```python
from build123d import *

# Parameters (mm, degrees)
F1_DEPTH = 0.3


with BuildPart() as f1:
    # F0 (on Top) → F1 (new body)
    with BuildSketch(Plane.XY):
        with BuildLine():
            ThreePointArc((68.445332, -5.526652), (68.785509, -6.832291), (68.9, -8.176652))
            Line((68.9, -8.176652), (102.9, -8.176652))
            Line((102.9, -8.176652), (102.9, 8.323348))
            Line((102.9, 8.323348), (87.9, 8.323348))
            ThreePointArc((87.9, 8.323348), (87.785509, 6.978988), (87.445332, 5.673348))
            ThreePointArc((87.445332, 5.673348), (79.95, 0.373348), (72.454668, 5.673348))
            ThreePointArc((72.454668, 5.673348), (72.114491, 6.978988), (72, 8.323348))
            Line((72, 8.323348), (49.9, 8.323348))
            ThreePointArc((49.9, 8.323348), (49.785509, 6.978988), (49.445332, 5.673348))
            ThreePointArc((49.445332, 5.673348), (41.95, 0.373348), (34.454668, 5.673348))
            ThreePointArc((34.454668, 5.673348), (34.114491, 6.978988), (34, 8.323348))
            Line((34, 8.323348), (0, 8.323348))
            Line((0, 8.323348), (0, -8.176652))
            Line((0, -8.176652), (15, -8.176652))
            ThreePointArc((15, -8.176652), (15.114491, -6.832291), (15.454668, -5.526652))
            ThreePointArc((15.454668, -5.526652), (22.95, -0.226652), (30.445332, -5.526652))
            ThreePointArc((30.445332, -5.526652), (30.785509, -6.832291), (30.9, -8.176652))
            Line((30.9, -8.176652), (53, -8.176652))
            ThreePointArc((53, -8.176652), (53.114491, -6.832291), (53.454668, -5.526652))
            ThreePointArc((53.454668, -5.526652), (60.95, -0.226652), (68.445332, -5.526652))
        make_face()
        with BuildLine():
            Line((15.454668, -5.526652), (30.445332, -5.526652))
            ThreePointArc((30.445332, -5.526652), (22.95, -0.226652), (15.454668, -5.526652))
        make_face()
        with BuildLine():
            ThreePointArc((34.454668, 5.673348), (41.95, 0.373348), (49.445332, 5.673348))
            Line((49.445332, 5.673348), (34.454668, 5.673348))
        make_face()
        with BuildLine():
            Line((53.454668, -5.526652), (68.445332, -5.526652))
            ThreePointArc((68.445332, -5.526652), (60.95, -0.226652), (53.454668, -5.526652))
        make_face()
        with BuildLine():
            ThreePointArc((72.454668, 5.673348), (79.95, 0.373348), (87.445332, 5.673348))
            Line((87.445332, 5.673348), (72.454668, 5.673348))
        make_face()
    extrude(amount=F1_DEPTH)


solid = f1.part
```
Can you work these out from the model? Positions are in its coordinate system, mm. Give positions to 0.01 mm unless a question says otherwise; leave off trailing zeros. Loops run counter-clockwise (first coordinate to the right, second up) from the corner with the lowest first, then second, coordinate; pieces in that order, holes last. Notation, with made-up numbers: M 27.5,57 L 82.5,57 A16 cw 82.5,70 Z; hole C 13.5,-11 d4. An arc over 180 degrees is marked long. Answer in a Markdown table with one row per item.
1. Suppose I cut it at B-B on x = 25.5. Write out the boundary of the cut face in (y, z), plus the area to 4 significant figures.
Taken from the geometry:
| item | result |
|---|---|
| outline | M -5.53,0 L 8.32,0 L 8.32,0.3 L -5.53,0.3 Z |
| area | 4.155 mm² |
2. Suppose I cut it at A-A on z = 0.15. Write out the boundary of the cut face in (x, y).
Taken from the geometry:
| item | result |
|---|---|
| outline | M 0,-8.18 L 15,-8.18 A7.95 cw 15.45,-5.53 L 30.45,-5.53 A7.95 cw 30.9,-8.18 L 53,-8.18 A7.95 cw 53.45,-5.53 L 68.45,-5.53 A7.95 cw 68.9,-8.18 L 102.9,-8.18 L 102.9,8.32 L 87.9,8.32 A7.95 cw 87.45,5.67 L 72.45,5.67 A7.95 cw 72,8.32 L 49.9,8.32 A7.95 cw 49.45,5.67 L 34.45,5.67 A7.95 cw 34,8.32 L 0,8.32 Z |
3. If I drill on line 1 along X through (y, z) = (7.75, 0.05); line 2 along X through (y, z) = (5.75, 0.25); line 3 along Y through (x, z) = (49, 0.15), over which ranges is the centre line in solid material (lowest first)?
Taken from the geometry:
| item | result |
|---|---|
| line 1 | x = 0 to 34.02, 49.88 to 72.02, 87.88 to 102.9 |
| line 2 | x = 0 to 34.43, 49.47 to 72.43, 87.47 to 102.9 |
| line 3 | y = -8.18 to 5.67 |
